Build history of the part. All positions in model axes, mm. Face numbers are marked on the shaded views. A direction names the side the tool comes from. Give positions to 0.01 mm unless a question says otherwise; leave off trailing zeros. Loops run counter-clockwise (first coordinate to the right, second up) from the corner with the lowest first, then second, coordinate; pieces in that order, holes last. Notation, with made-up numbers: (40, 55.5) -> (62, 55.5) arc R27 cw to (62, 73.5) -> close; hole circle Ø8 at (12, 81.25). An arc over 180 degrees is marked (long way). Answer in a Markdown table with one row per item. Add a question column.
from build123d import *

# Parameters (mm, degrees)
SKETCH1_W              = 60
SKETCH1_H              = 30
BASE_FLANGE1_DEPTH     = 1
SKETCHED_START         = -15
SKETCHED_BEND1_DEPTH   = 30
SKETCHED_BEND1_2_DEPTH = 30
SKETCHED_BEND2_DEPTH   = 30
SKETCHED_BEND2_2_DEPTH = 30
CUT_EXTRUDE1_DEPTH     = 10
CUT_EXTRUDE2_DEPTH     = 10
FILLET1_R              = 3


# Read off the part's stored shape, not the designer's step: Sketched Bend1, Sketched Bend2
# Sheet-metal steps are written as plain solids
with BuildPart() as part:
    # Sketch1 → Base-Flange1 (new body)
    with BuildSketch(Plane.XY):
        Rectangle(SKETCH1_W, SKETCH1_H)
    extrude(amount=-BASE_FLANGE1_DEPTH)

    # Sketched Bend1 outline → Sketched Bend1 (cut)
    with BuildSketch(Plane(origin=(0, 0, 0), x_dir=(1, 0, 0), z_dir=(0, 1, 0)).offset(SKETCHED_START)):
        with BuildLine():
            Line((-30, 0), (9.398582279, 0))
            ThreePointArc((9.398582279, 0), (10.039397205, 0.728828115), (10.971223369, 1))
            Line((10.971223369, 1), (-30, 1))
            Line((-30, 1), (-30, 0))
        make_face()
    extrude(amount=SKETCHED_BEND1_DEPTH, mode=Mode.SUBTRACT)

    # Sketched Bend1 2 outline → Sketched Bend1 2 (add)
    with BuildSketch(Plane(origin=(0, 0, 0), x_dir=(1, 0, 0), z_dir=(0, 1, 0)).offset(SKETCHED_START)):
        with BuildLine():
            ThreePointArc((9.398582279, 0), (9.276108612, -0.359286442), (9.234623369, -0.7366))
            Line((9.234623369, -0.7366), (9.234623369, -39.765376631))
            Line((9.234623369, -39.765376631), (10.234623369, -39.765376631))
            Line((10.234623369, -39.765376631), (10.234623369, -0.7366))
            ThreePointArc((10.234623369, -0.7366), (10.450368514, -0.215745145), (10.971223369, 0))
            Line((10.971223369, 0), (9.398582279, 0))
        make_face()
    extrude(amount=SKETCHED_BEND1_2_DEPTH)

    # Sketched Bend2 outline → Sketched Bend2 (cut)
    with BuildSketch(Plane(origin=(0, 0, 0), x_dir=(1, 0, 0), z_dir=(0, 1, 0)).offset(SKETCHED_START)):
        with BuildLine():
            Line((9.234623369, -0.7366), (9.234623369, -19.16395891))
            ThreePointArc((9.234623369, -19.16395891), (9.963451484, -19.804773836), (10.234623369, -20.7366))
            Line((10.234623369, -20.7366), (10.234623369, -0.7366))
            ThreePointArc((10.234623369, -0.7366), (10.450368514, -0.215745145), (10.971223369, 0))
            Line((10.971223369, 0), (30, 0))
            Line((30, 0), (30, 1))
            Line((30, 1), (10.971223369, 1))
            ThreePointArc((10.971223369, 1), (9.743261733, 0.491361636), (9.234623369, -0.7366))
        make_face()
    extrude(amount=SKETCHED_BEND2_DEPTH, mode=Mode.SUBTRACT)

    # Sketched Bend2 2 outline → Sketched Bend2 2 (add)
    with BuildSketch(Plane(origin=(0, 0, 0), x_dir=(1, 0, 0), z_dir=(0, 1, 0)).offset(SKETCHED_START)):
        with BuildLine():
            ThreePointArc((-11.296129893, -18.2634), (-10.78749153, -19.491361636), (-9.559529893, -20))
            Line((-9.559529893, -20), (8.498023369, -20))
            ThreePointArc((8.498023369, -20), (9.018878224, -20.215745145), (9.234623369, -20.7366))
            Line((9.234623369, -20.7366), (9.234623369, -19.16395891))
            ThreePointArc((9.234623369, -19.16395891), (8.875336927, -19.041485243), (8.498023369, -19))
            Line((8.498023369, -19), (-9.559529893, -19))
            ThreePointArc((-9.559529893, -19), (-10.080384748, -18.784254855), (-10.296129893, -18.2634))
            Line((-10.296129893, -18.2634), (-10.296129893, 0.765376631))
            Line((-10.296129893, 0.765376631), (-11.296129893, 0.765376631))
            Line((-11.296129893, 0.765376631), (-11.296129893, -18.2634))
        make_face()
    extrude(amount=SKETCHED_BEND2_2_DEPTH)

    # Sketch8 → Cut-Extrude1 (cut)
    with BuildSketch(Plane(origin=(10.234623369, 0, 0), x_dir=(0, 0, -1), z_dir=(1, 0, 0))):
        with BuildLine():
            Line((-34.765376631, 11.5), (-29.765376631, 11.5))
            ThreePointArc((-29.765376631, 11.5), (-27.265376631, 9), (-29.765376631, 6.5))
            Line((-29.765376631, 6.5), (-34.765376631, 6.5))
            ThreePointArc((-34.765376631, 6.5), (-37.265376631, 9), (-34.765376631, 11.5))
        make_face()
        with BuildLine():
            Line((-34.765376631, -6.5), (-29.765376631, -6.5))
            ThreePointArc((-29.765376631, -6.5), (-27.265376631, -9), (-29.765376631, -11.5))
            Line((-29.765376631, -11.5), (-34.765376631, -11.5))
            ThreePointArc((-34.765376631, -11.5), (-37.265376631, -9), (-34.765376631, -6.5))
        make_face()
    extrude(amount=-CUT_EXTRUDE1_DEPTH, mode=Mode.SUBTRACT)

    # Sketch9 → Cut-Extrude2 (cut)
    with BuildSketch(Plane(origin=(-10.296129893, 0, 0), x_dir=(0, 0, -1), z_dir=(1, 0, 0))):
        with BuildLine():
            Line((-9.234623369, 11.5), (-4.234623369, 11.5))
            ThreePointArc((-4.234623369, 11.5), (-1.734623369, 9), (-4.234623369, 6.5))
            Line((-4.234623369, 6.5), (-9.234623369, 6.5))
            ThreePointArc((-9.234623369, 6.5), (-11.734623369, 9), (-9.234623369, 11.5))
        make_face()
        with BuildLine():
            Line((-9.234623369, -6.5), (-4.234623369, -6.5))
            ThreePointArc((-4.234623369, -6.5), (-1.734623369, -9), (-4.234623369, -11.5))
            Line((-4.234623369, -11.5), (-9.234623369, -11.5))
            ThreePointArc((-9.234623369, -11.5), (-11.734623369, -9), (-9.234623369, -6.5))
        make_face()
    extrude(amount=-CUT_EXTRUDE2_DEPTH, mode=Mode.SUBTRACT)

    # Fillet1
    fillet1_edges = [part.edges().sort_by_distance(p)[0] for p in [
        (-10.796129893, 15, -0.765376631),
        (-10.796129893, -15, -0.765376631),
        (9.734623369, -15, 39.765376631),
        (9.734623369, 15, 39.765376631),
    ]]
    fillet(fillet1_edges, radius=FILLET1_R)


solid = part.part
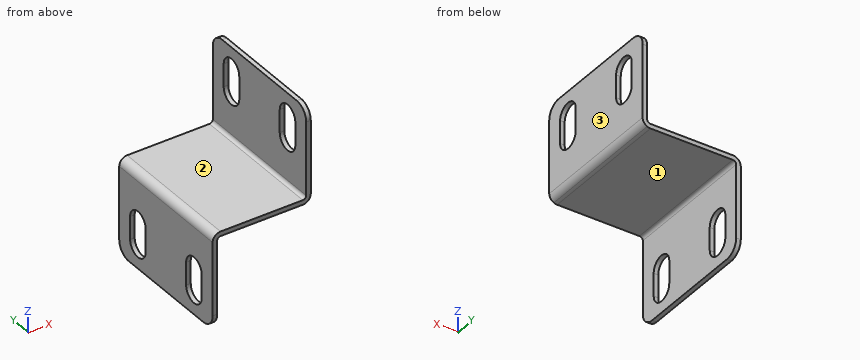
(1) Saw through at C-C, the plane x = 5.5. List the corners of the cut face in (y, z), then the cut area to 3 significant figures.
(2) Wall check: line 1 along X through (y, z) = (1.75, 17); line 2 along Z through (x, y) = (-3, 6.5); line 3 along X through (y, z) = (2, 26.5). Give the ranges that are in metal, low to high. Write a range as from..to.
(3) 3-axis set-ups, long thin cutter, end or side, ignore diameter. For the marked faces 1, 2 and 3: which of +Z, -Z, +X, -X, +Y, -Y reach the whole face in a straight line?
(4) Saw through at B-B, the plane z = 23. List the corners of the cut face in (x, y).
(5) Flat gauge pins, fed straight in: pin 1 Ø5.5 at (x, y) = (0.5, 1) entering from +Z; pin 2 Ø1 at (y, z) = (-4, 20) entering from +X; pin 3 Ø2 at (y, z) = (9.5, 15.5) entering from +X. Where does each tip first touch, or does it go through?
(6) Saw through at A-A, the plane y = -9. List the corners of the cut face in (x, z).
Worked answers:
| question | item | result |
|---|---|---|
| 1 | outline | (-15, 19) -> (15, 19) -> (15, 20) -> (-15, 20) -> close |
| 1 | area | 30.0 mm^2 |
| 2 | line 1 | -11.3..-10.3 |
| 2 | line 2 | 19..20 |
| 2 | line 3 | 9.23..10.23 |
| 3 | face 1 | -Z, +X, +Y, -Y |
| 3 | face 2 | +Z, -X, +Y, -Y |
| 3 | face 3 | +Z, -Z, +X, +Y, -Y |
| 4 | outline | (9.23, -15) -> (10.23, -15) -> (10.23, 15) -> (9.23, 15) -> close |
| 5 | pin 1 | z = 20 |
| 5 | pin 2 | x = 10.22 |
| 5 | pin 3 | x = -10.3 |
| 6 | outline | (-11.3, -0.77) -> (-10.3, -0.77) -> (-10.3, 1.73) -> (-11.3, 1.73) -> close; (-11.3, 11.73) -> (-10.3, 11.73) -> (-10.3, 18.26) arc R0.74 cw to (-9.56, 19) -> (8.5, 19) arc R1.74 ccw to (10.23, 20.74) -> (10.23, 27.27) -> (9.23, 27.27) -> (9.23, 20.74) arc R0.74 cw to (8.5, 20) -> (-9.56, 20) arc R1.74 ccw to (-11.3, 18.26) -> close; (9.23, 37.27) -> (10.23, 37.27) -> (10.23, 39.77) -> (9.23, 39.77) -> close |
